from build123d import *

# Parameters (mm, degrees)
F1_DEPTH = 250.825
F3_DEPTH = 664.211


with BuildPart() as f1:
    # F0 (on Top) → F1 (new body)
    with BuildSketch(Plane.XY):
        with BuildLine():
            ThreePointArc((0, -224.79), (0.743949, -226.586051), (2.54, -227.33))
            Line((2.54, -227.33), (661.67, -227.33))
            ThreePointArc((661.67, -227.33), (663.466051, -226.586051), (664.21, -224.79))
            Line((664.21, -224.79), (664.21, 0))
            Line((664.21, 0), (662.305, 0))
            Line((662.305, 0), (662.305, -225.425))
            Line((662.305, -225.425), (1.905, -225.425))
            Line((1.905, -225.425), (1.905, 0))
            Line((1.905, 0), (0, 0))
            Line((0, 0), (0, -224.79))
        make_face()
    extrude(amount=F1_DEPTH)

    # F2 (on face) → F3 (cut, through all)
    with BuildSketch(Plane.YZ.offset(664.21)):
        with BuildLine():
            ThreePointArc((-7.9248, 228.6), (-6.064928, 224.109872), (-1.5748, 222.25))
            Line((-1.5748, 222.25), (0, 222.25))
            Line((0, 222.25), (0, 250.825))
            Line((0, 250.825), (-7.9248, 250.825))
            Line((-7.9248, 250.825), (-7.9248, 228.6))
        make_face()
    extrude(amount=-F3_DEPTH, mode=Mode.SUBTRACT)


solid = f1.part
The listing builds one solid part. Answer for the finished solid, in the listing's coordinates (mm). A direction names the side the tool comes from. Give positions to 0.01 mm unless a question says otherwise; leave off trailing zeros. Write each loop counter-clockwise with the first axis right and the second up, starting at its lowest first coordinate (ties: lowest second). Pieces come first, ordered by that corner, then holes. Notation, with made-up numbers: (-2.75, -39) - (23.25, -39) arc R16 ccw to (23.25, -22) - close; hole circle Ø11 at (14.25, 70). An arc over 180 degrees is marked (long way). Use a Markdown table: item, result.
1. Section C-C on x = 70 is taken. Write down the section's boundary in (y, z) (3 decimals), plus the area to 3 significant figures.
Values follow:
| item | result |
|---|---|
| outline | (-227.33, 0) - (-225.425, 0) - (-225.425, 250.825) - (-227.33, 250.825) - close |
| area | 478 mm² |
2. A tool of negligible diameter and unlimited length cuts with its end or side. For faces 1 (the flat face through (327, -227.33, 124)), 2 (the flat face through (1.905, -114, 124)), from which of +Z, -Z, +X, -X, +Y, -Y can it reach the whole face along a straight path? Write none if from no direction.
Values follow:
| item | result |
|---|---|
| face 1 | +Z, -Z, +X, -X, -Y |
| face 2 | +Z, -Z, +Y |
3. Section B-B on z = 28.5 is taken. Write down the section's boundary in (x, y) (3 decimals), plus the area to 3 significant figures.
Values follow:
| item | result |
|---|---|
| outline | (0, -224.79) arc R2.54 ccw to (2.54, -227.33) - (661.67, -227.33) arc R2.54 ccw to (664.21, -224.79) - (664.21, 0) - (662.305, 0) - (662.305, -225.425) - (1.905, -225.425) - (1.905, 0) - (0, 0) - close |
| area | 2,120 mm² |
4. For a pull along X with two mould halves and no side action, classify faces 3 (the flat face through (662.305, -111, 124)), 4 (the flat face through (0, -111, 124)), 5 (the flat face through (337, -225.425, 124)), 6 (the flat face through (664.21, -114, 124)) as released by +X, released by -X, zero draft, split by the parting line, or undercut.
Values follow:
| item | result |
|---|---|
| face 3 | undercut |
| face 4 | released by -X |
| face 5 | undercut |
| face 6 | released by +X |
5. Find the intervals of material crossed by probe 1 along X at (y, z) = (-159, 24) (3 decimals); probe 2 along Y at (x, z) = (202, 170) (3 decimals), in increasing order. Write a range as from..to.
Values follow:
| item | result |
|---|---|
| probe 1 | x = 0..1.905, 662.305..664.21 |
| probe 2 | y = -227.33..-225.425 |
6. Each of these flat-tipped pins is pushed along its axis until it touches: P1, Ø3, axis at x = 579, z = 170, coming from the +Y side (3 decimals); P2, Ø1.3, axis at x = 0.5, y = -1, coming from the +Z side; P3, Ø1, axis at x = 663.5, z = 237, coming from the +Y side. Where does it stop, or does it pass through?
Values follow:
| item | result |
|---|---|
| P1 | stops at y = -225.425 |
| P2 | stops at z = 222.25 |
| P3 | stops at y = -7.92 |
7. Section A-A on y = -176.5 is taken. Write down the section's boundary in (x, z) (3 decimals).
Values follow:
| item | result |
|---|---|
| outline | (0, 0) - (1.905, 0) - (1.905, 250.825) - (0, 250.825) - close; (662.305, 0) - (664.21, 0) - (664.21, 250.825) - (662.305, 250.825) - close |
